```python
from build123d import *

# Parameters (mm, degrees)
F0_W     = 76.6426213086
F0_H     = 55.3530044854
F1_DEPTH = 25.4
F2_W     = 76.6426213086
F2_H     = 9.5973666757
F3_DEPTH = 20.32
F2_H_2   = 8.4236329421
F4_DEPTH = 15.24
F2_H_3   = 9.6555026248
F5_DEPTH = 10.16
F2_H_4   = 8.3485189825
F6_DEPTH = 10.16
F2_H_5   = 8.8109364733
F7_DEPTH = 15.24
F2_H_6   = 10.5170467868
F8_DEPTH = 20.32


with BuildPart() as f1:
    # F0 (on Top) → F1 (new body)
    with BuildSketch(Plane.XY):
        with Locations((-0.0834930688, -1.8811021)):
            Rectangle(F0_W, F0_H)
    extrude(amount=F1_DEPTH)

    # F2 (on face) → F3 (cut)
    with BuildSketch(Plane.XY.offset(25.4)):
        with Locations((-0.0834930688, -24.7589210048)):
            Rectangle(F2_W, F2_H)
    extrude(amount=-F3_DEPTH, mode=Mode.SUBTRACT)

    # F2 (on face) → F4 (cut)
    with BuildSketch(Plane.XY.offset(25.4)):
        with Locations((-0.0834930688, -15.7484211959)):
            Rectangle(F2_W, F2_H_2)
    extrude(amount=-F4_DEPTH, mode=Mode.SUBTRACT)

    # F2 (on face) → F5 (cut)
    with BuildSketch(Plane.XY.offset(25.4)):
        with Locations((-0.0834930688, -6.7088534124)):
            Rectangle(F2_W, F2_H_3)
    extrude(amount=-F5_DEPTH, mode=Mode.SUBTRACT)

    # F2 (on face) → F6 (cut)
    with BuildSketch(Plane.XY.offset(25.4)):
        with Locations((-0.0834930688, 2.2931573913)):
            Rectangle(F2_W, F2_H_4)
    extrude(amount=-F6_DEPTH, mode=Mode.SUBTRACT)

    # F2 (on face) → F7 (cut)
    with BuildSketch(Plane.XY.offset(25.4)):
        with Locations((-0.0834930688, 10.8728851192)):
            Rectangle(F2_W, F2_H_5)
    extrude(amount=-F7_DEPTH, mode=Mode.SUBTRACT)

    # F2 (on face) → F8 (cut)
    with BuildSketch(Plane.XY.offset(25.4)):
        with Locations((-0.0834930688, 20.5368767492)):
            Rectangle(F2_W, F2_H_6)
    extrude(amount=-F8_DEPTH, mode=Mode.SUBTRACT)


solid = f1.part
```
Can you work these out from the model? Positions are in its coordinate system, mm. A direction names the side the tool comes from. Give positions to 0.01 mm unless a question says otherwise; leave off trailing zeros. Loops run counter-clockwise (first coordinate to the right, second up) from the corner with the lowest first, then second, coordinate; pieces in that order, holes last. Notation, with made-up numbers: M 65.25,76 L 115.25,76 A35 cw 115.25,111 Z; hole C 88.25,87.5 d1. An arc over 180 degrees is marked long. One line per question, with ' | ' between items. Start each with the question number.
Q1. For faces 1 (the flat face through (-1, 6.467, 13)), 2 (the flat face through (38.238, -2, 6)), 3 (the flat face through (-1, -19.96, 8)), which set-ups out of +Z, -Z, +X, -X, +Y, -Y let a thin tool reach every point of the face, with its end or its side?
Q2. For pin 1 Ø6.5 at (x, y) = (-2.5, -16.5) entering from +Z; pin 2 Ø2.5 at (x, z) = (-16.5, 12) entering from -Y; pin 3 Ø4 at (x, z) = (17, 13) entering from +Y, each with a flat end and sliding along its axis, tell me the tip position at first contact or that it passes through.
Q3. If we section it at C-C (y = -12.5): Please give me the cut outline in (x, z), plus the area to 3 significant figures.
Q4. If we section it at B-B (z = 11): Please give me the cut outline in (x, y), plus the area to 3 significant figures.
Q5. If we section it at A-A (x = -6.5): Please give me the cut outline in (y, z).
Q6. If I drill on line 1 (Y direction, x = -20.5, z = 9.5); line 2 (Z direction, x = 0, y = -19.5); line 3 (Z direction, x = 30, y = 22), over which ranges is the centre line in solid material (lowest first)? Write a range as from..to.
Computed:
1) face 1: +Z, +X, -X, +Y | face 2: +Z, -Z, +X, +Y, -Y | face 3: +Z, +X, -X, -Y
2) pin 1: stops at z = 10.16 | pin 2: stops at y = -11.54 | pin 3: stops at y = 6.47
3) outline: M -38.4,0 L 38.24,0 L 38.24,10.16 L -38.4,10.16 Z | area: 779 mm²
4) outline: M -38.4,-11.54 L 38.24,-11.54 L 38.24,6.47 L -38.4,6.47 Z | area: 1,380 mm²
5) outline: M -29.56,0 L 25.8,0 L 25.8,5.08 L 15.28,5.08 L 15.28,10.16 L 6.47,10.16 L 6.47,15.24 L -11.54,15.24 L -11.54,10.16 L -19.96,10.16 L -19.96,5.08 L -29.56,5.08 Z
6) line 1: y = -19.96..15.28 | line 2: z = 0..10.16 | line 3: z = 0..5.08
